from build123d import *

# Parameters (mm, degrees)
SKETCH1_W           = 200
SKETCH1_H           = 213
SKETCH1_R           = 9.5
BOSS_EXTRUDE1_DEPTH = 25
SKETCH2_R           = 35
SKETCH2_R_2         = 19.03
BOSS_EXTRUDE2_DEPTH = 114
SKETCH3_R           = 35
SKETCH3_R_2         = 19.03
BOSS_EXTRUDE3_DEPTH = 51
CUT_EXTRUDE1_DEPTH  = 51
BOSS_EXTRUDE4_START = 76
BOSS_EXTRUDE4_DEPTH = 76
SKETCH5_W           = 19
SKETCH5_H           = 46.369491486
BOSS_EXTRUDE5_DEPTH = 17
BOSS_EXTRUDE6_START = -83
SKETCH6_W           = 19
SKETCH6_H           = 46.471332412
BOSS_EXTRUDE6_DEPTH = 83
FILLET3_R           = 3


with BuildPart() as part:
    # Sketch1 → Boss-Extrude1 (new body)
    with BuildSketch(Plane(origin=(0, 0, 0), x_dir=(1, 0, 0), z_dir=(0, 1, 0))):
        Rectangle(SKETCH1_W, SKETCH1_H)
        with Locations(Location((68, -49.5, 0), (0, 0, 270))):
            Circle(SKETCH1_R, mode=Mode.SUBTRACT)
        with Locations(Location((68, -87.5, 0), (0, 0, 270))):
            Circle(SKETCH1_R, mode=Mode.SUBTRACT)
        with Locations(Location((-84, -49.5, 0), (0, 0, 270))):
            Circle(SKETCH1_R, mode=Mode.SUBTRACT)
        with Locations(Location((-84, -87.5, 0), (0, 0, 270))):
            Circle(SKETCH1_R, mode=Mode.SUBTRACT)
    extrude(amount=BOSS_EXTRUDE1_DEPTH)

    # Sketch4 → Cut-Extrude1 (cut)
    with BuildSketch(Plane(origin=(0, 25, 0), x_dir=(1, 0, 0), z_dir=(0, 1, 0))):
        with BuildLine():
            Line((-100, 106.5), (-100, -4.5))
            Line((-100, -4.5), (19, -4.5))
            ThreePointArc((19, -4.5), (50.819805153, 8.680194847), (64, 40.5))
            Line((64, 40.5), (64, 106.5))
            Line((64, 106.5), (-100, 106.5))
        make_face()
    extrude(amount=-CUT_EXTRUDE1_DEPTH, mode=Mode.SUBTRACT)



with BuildPart() as body_2:
    # Sketch2 → Boss-Extrude2 (new body)
    with BuildSketch(Plane.XY.offset(106.5)):
        with Locations((-17, 102)):
            Circle(SKETCH2_R)
        with Locations((-17, 102)):
            Circle(SKETCH2_R_2, mode=Mode.SUBTRACT)
    extrude(amount=-BOSS_EXTRUDE2_DEPTH)


with BuildPart() as body_3:
    # Sketch3 → Boss-Extrude3 (new body)
    with BuildSketch(Plane(origin=(100, 0, 0), x_dir=(0, 0, -1), z_dir=(1, 0, 0))):
        with Locations((71.5, 102)):
            Circle(SKETCH3_R)
        with Locations((71.5, 102)):
            Circle(SKETCH3_R_2, mode=Mode.SUBTRACT)
    extrude(amount=-BOSS_EXTRUDE3_DEPTH)


with BuildPart() as part_1:
    add(part.part)

    add(body_2.part)  # Boss-Extrude4 merges body 2

    add(body_3.part)  # Boss-Extrude4 merges body 3
    # Sketch4<3> → Boss-Extrude4 (add)
    with BuildSketch(Plane(origin=(0, 25, 0), x_dir=(1, 0, 0), z_dir=(0, 1, 0)).offset(BOSS_EXTRUDE4_START)):
        with BuildLine():
            Line((-100, -4.5), (-100, -23.5))
            Line((-100, -23.5), (19, -23.5))
            ThreePointArc((19, -23.5), (64.254833996, -4.754833996), (83, 40.5))
            Line((83, 40.5), (83, 106.5))
            Line((83, 106.5), (64, 106.5))
            Line((64, 106.5), (64, 40.5))
            ThreePointArc((64, 40.5), (50.819805153, 8.680194847), (19, -4.5))
            Line((19, -4.5), (-100, -4.5))
        make_face()
    extrude(amount=-BOSS_EXTRUDE4_DEPTH)

    # Sketch5 → Boss-Extrude5 (add)
    with BuildSketch(Plane(origin=(100, 0, 0), x_dir=(0, 0, -1), z_dir=(1, 0, 0))):
        with Locations((71.5, 48.184745743)):
            Rectangle(SKETCH5_W, SKETCH5_H)
    extrude(amount=-BOSS_EXTRUDE5_DEPTH)

    # Sketch6 → Boss-Extrude6 (add)
    with BuildSketch(Plane.XY.offset(106.5).offset(BOSS_EXTRUDE6_START)):
        with Locations((-17, 48.235666206)):
            Rectangle(SKETCH6_W, SKETCH6_H)
    extrude(amount=BOSS_EXTRUDE6_DEPTH)

    # Fillet3
    fillet3_edges = [part_1.edges().sort_by_distance(p)[0] for p in [
        (83, 63, -106.5),
        (-7.5, 46.656974737, 106.5),
        (-26.5, 46.656974737, 106.5),
        (-100, 25, 65),
        (18.492855685, 101, 23.5),
        (83, 25, -51.25),
        (5.75, 25, 23.5),
        (100, 25, -93.75),
        (91.5, 25, -106.5),
        (83, 25, -93.75),
        (83, 46.656974737, -81),
        (100, 46.656974737, -81),
        (100, 46.656974737, -62),
        (83, 46.656974737, -62),
        (62.82302176, 101, 6.142713941),
        (64.254833996, 25, 4.754833996),
        (100, 25, 22.25),
        (46.25, 25, 106.5),
        (-7.5, 46.656974737, 23.5),
        (-7.5, 25, 65),
        (-63.25, 25, 106.5),
        (-63.25, 25, 23.5),
        (-26.5, 25, 65),
        (-26.5, 46.656974737, 23.5),
        (-100, 63, 23.5),
        (-75.992855685, 101, 23.5),
    ]]
    fillet(fillet3_edges, radius=FILLET3_R)


solid = part_1.part
CAD build for the part. Positions are in the model's coordinates, mm. A direction names the side the tool comes from. Give positions to 0.01 mm unless a question says otherwise; leave off trailing zeros. Order: outer loops, then holes, each group sorted by start corner. A loop starts at its lowest first (then second) coordinate and runs counter-clockwise, first axis right, second up. Notation, with made-up numbers: (-17.5, 18.5) - (-8.5, 18.5) arc R22 ccw to (-8.5, 47.5) - close; hole circle Ø7 at (-9.75, -36). An arc over 180 degrees is marked (long way). Answer in a Markdown table with one row per item.
1. Saw through at B-B, the plane x = -84. Give the cut face in (y, z).
Data:
| item | result |
|---|---|
| outline | (0, 4.5) - (101, 4.5) - (101, 20.5) arc R3 ccw to (98, 23.5) - (28, 23.5) arc R3 cw to (25, 26.5) - (25, 40) - (0, 40) - close; (0, 59) - (25, 59) - (25, 78) - (0, 78) - close; (0, 97) - (25, 97) - (25, 103.5) arc R3 ccw to (22, 106.5) - (0, 106.5) - close |
2. Tool access for faces 5 (the flat face through (64, 94, -72)), 6 (the flat face through (-64, 25, 64)), 7 (the flat face through (91, 25, -92)): list every direction of +Z, -Z, +X, -X, +Y, -Y with a clear straight run to the whole face (end or side of a thin tool).
Data:
| item | result |
|---|---|
| face 5 | -X |
| face 6 | +Z, -X |
| face 7 | -Z, +X |
3. Saw through at C-C, the plane x = -18. Give the cut face in (y, z), plus the area to 3 significant figures.
Data:
| item | result |
|---|---|
| outline | (0, 4.5) - (67.01, 4.5) - (67.01, -7.5) - (83, -7.5) - (83, 4.5) - (101, 4.5) - (101, 23.5) - (83, 23.5) - (83, 106.5) - (0, 106.5) - close; (121, -7.5) - (136.99, -7.5) - (136.99, 106.5) - (121, 106.5) - close |
| area | 10,800 mm² |
4. Pull direction X, two halves, no side cores. Call faces 1 (the cylindrical face through (76.01, 12.32, 54.61)), 2 (the flat face through (49, 87, -87)), 3 (the cylindrical face through (51.168, 51.207, -9.032)), 4 (the flat face through (-7.5, 48, 64)): pulls with the +X half, pulls with the -X half, needs draft (parallel to the pull), parting line crosses it, or undercut.
Data:
| item | result |
|---|---|
| face 1 | undercut |
| face 2 | pulls with the -X half |
| face 3 | undercut |
| face 4 | pulls with the +X half |
5. Saw through at D-D, the plane y = 50.5. Give the cut face in (x, z), plus the area to 3 significant figures.
Data:
| item | result |
|---|---|
| outline | (-100, 4.5) - (19, 4.5) arc R45 cw to (64, -40.5) - (64, -106.5) - (80, -106.5) arc R3 ccw to (83, -103.5) - (83, -84) arc R3 cw to (86, -81) - (97, -81) arc R3 ccw to (100, -78) - (100, -65) arc R3 ccw to (97, -62) - (86, -62) arc R3 cw to (83, -59) - (83, -40.5) arc R64 ccw to (19, 23.5) - (-4.5, 23.5) arc R3 cw to (-7.5, 26.5) - (-7.5, 103.5) arc R3 ccw to (-10.5, 106.5) - (-23.5, 106.5) arc R3 ccw to (-26.5, 103.5) - (-26.5, 26.5) arc R3 cw to (-29.5, 23.5) - (-97, 23.5) arc R3 ccw to (-100, 20.5) - close |
| area | 7,040 mm² |
6. Flat gauge pins, fed straight in: pin 1 (5 mm diameter, centred on x = -47.5, z = 24.5, fed in from -Y); pin 2 (5.5 mm diameter, centred on x = -16, y = 96, fed in from -Z); pin 3 (15.5 mm diameter, centred on y = 65, z = -96, fed in from +X); pin 4 (7 mm diameter, centred on x = 9, y = 53.5, fed in from +Z). Where does each tip first touch, or does it go through?
Data:
| item | result |
|---|---|
| pin 1 | stops at y = 0 |
| pin 2 | stops at z = 4.5 |
| pin 3 | stops at x = 83 |
| pin 4 | stops at z = 23.5 |
7. Probe probe 1 along X at (y, z) = (10, 87); probe 2 along X at (y, z) = (89, -83); probe 3 along Y at (x, z) = (-17, 20.5). List the from-to ranges inside material, lowest first. Write a range as [from, to].
Data:
| item | result |
|---|---|
| probe 1 | x = [-100, -93.49], [-74.51, 58.51], [77.49, 100] |
| probe 2 | x = [64, 83] |
| probe 3 | y = [0, 101], [121.03, 137] |
8. Saw through at A-A, the plane z = 87.5. Give the cut face in (x, y).
Data:
| item | result |
|---|---|
| outline | (-100, 0) - (-93.5, 0) - (-93.5, 25) - (-97, 25) arc R3 ccw to (-100, 22) - close; (-74.5, 0) - (58.5, 0) - (58.5, 25) - (-4.5, 25) arc R3 cw to (-7.5, 28) - (-7.5, 68.31) arc R35 ccw (long way) to (-26.5, 68.31) - (-26.5, 28) arc R3 cw to (-29.5, 25) - (-74.5, 25) - close; (77.5, 0) - (100, 0) - (100, 22) arc R3 ccw to (97, 25) - (77.5, 25) - close; hole circle Ø38.06 at (-17, 102) |
